Verification items for the finished model (mm, model axes). A direction names the side the tool comes from. Round coordinates to 2 decimals unless told otherwise and drop trailing zeros. Loops run counter-clockwise (first coordinate to the right, second up) from the corner with the lowest first, then second, coordinate; pieces in that order, holes last. Notation, with made-up numbers: (70, 36) -> (94, 36) arc R25 cw to (94, 67) -> close; hole circle Ø6 at (-20, -20). An arc over 180 degrees is marked (long way). Write item = value, one per line.
```python
from build123d import *

# Parameters (mm, degrees)
F1_DEPTH = 38.1
F3_DEPTH = 12.7
F5_DEPTH = 12.7


with BuildPart() as f1:
    # F0 (on Front) → F1 (new body)
    with BuildSketch(Plane.XZ):
        Polygon((-50.8, 0), (0, 0), (0, 19.05), (-12.7, 19.05), (-12.7, 6.35), (-44.45, 6.35), (-44.45, 19.05), (-50.8, 19.05), align=None)
    extrude(amount=F1_DEPTH)

    # F2 (on face) → F3 (cut)
    with BuildSketch(Plane.XY.offset(19.05)):
        Polygon((-12.7, -38.1), (0, -12.7), (0, 0), (-12.7, 0), align=None)
    extrude(amount=-F3_DEPTH, mode=Mode.SUBTRACT)

    # F4 (on face) → F5 (join)
    with BuildSketch(Plane.XY.offset(6.35)):
        Polygon((-19.05, 0), (-44.45, 0), (-44.45, -38.1), align=None)
    extrude(amount=F5_DEPTH)


solid = f1.part
```
(1) Sectioned sample at B-B, the plane x = -5.5. Record the cut outline in (y, z).
Filled sheet:
outline = (-38.1, 0) -> (0, 0) -> (0, 6.35) -> (-23.7, 6.35) -> (-23.7, 19.05) -> (-38.1, 19.05) -> close
(2) Material ranges on probe 1 along Z at (x, y) = (-34, -24); probe 2 along X at (y, z) = (-17, 13.5), recorded low to high. Write a range as from..to.
Filled sheet:
probe_1 = 0..6.35
probe_2 = -50.8..-30.38, -2.15..0
(3) Sectioned sample at A-A, the plane z = 7.25. Record the cut outline in (x, y).
Filled sheet:
outline = (-50.8, -38.1) -> (-44.45, -38.1) -> (-19.05, 0) -> (-50.8, 0) -> close; (-12.7, -38.1) -> (0, -38.1) -> (0, -12.7) -> close
(4) Sectioned sample at C-C, the plane y = -23.5. Record the cut outline in (x, z).
Filled sheet:
outline = (-50.8, 0) -> (0, 0) -> (0, 19.05) -> (-5.4, 19.05) -> (-5.4, 6.35) -> (-34.72, 6.35) -> (-34.72, 19.05) -> (-50.8, 19.05) -> close
(5) Go/stop test with a flat-tipped pin: pin 1 Ø3 at (x, y) = (-15.5, -16.5) entering from +Z. Record where the tip stops, or that it passes through.
Filled sheet:
pin_1 = 6.35
(6) Sectioned sample at D-D, the plane x = -12. Record the cut outline in (y, z).
Filled sheet:
outline = (-38.1, 0) -> (0, 0) -> (0, 6.35) -> (-36.7, 6.35) -> (-36.7, 19.05) -> (-38.1, 19.05) -> close
(7) Set-up check for faces 1 (the face through (-39, -15, 19.05)), 2 (the face through (-18, -19, 6.35)): record each of +Z, -Z, +X, -X, +Y, -Y from which the full face is reachable in a straight line by a thin tool's end or side.
Filled sheet:
face_1 = +Z, +X, -X, +Y, -Y
face_2 = +Z
(8) Draft check along X on faces 3 (the face through (-50.8, -19, 10)), 4 (the face through (-6.44, -25.58, 12.79)), 5 (the face through (-3, -31, 19.05)), 6 (the face through (-31.93, -19.32, 12.61)). Enter one of: released by +X, released by -X, zero draft, split by the parting line, or undercut.
Filled sheet:
face_3 = released by -X
face_4 = undercut
face_5 = zero draft
face_6 = undercut
